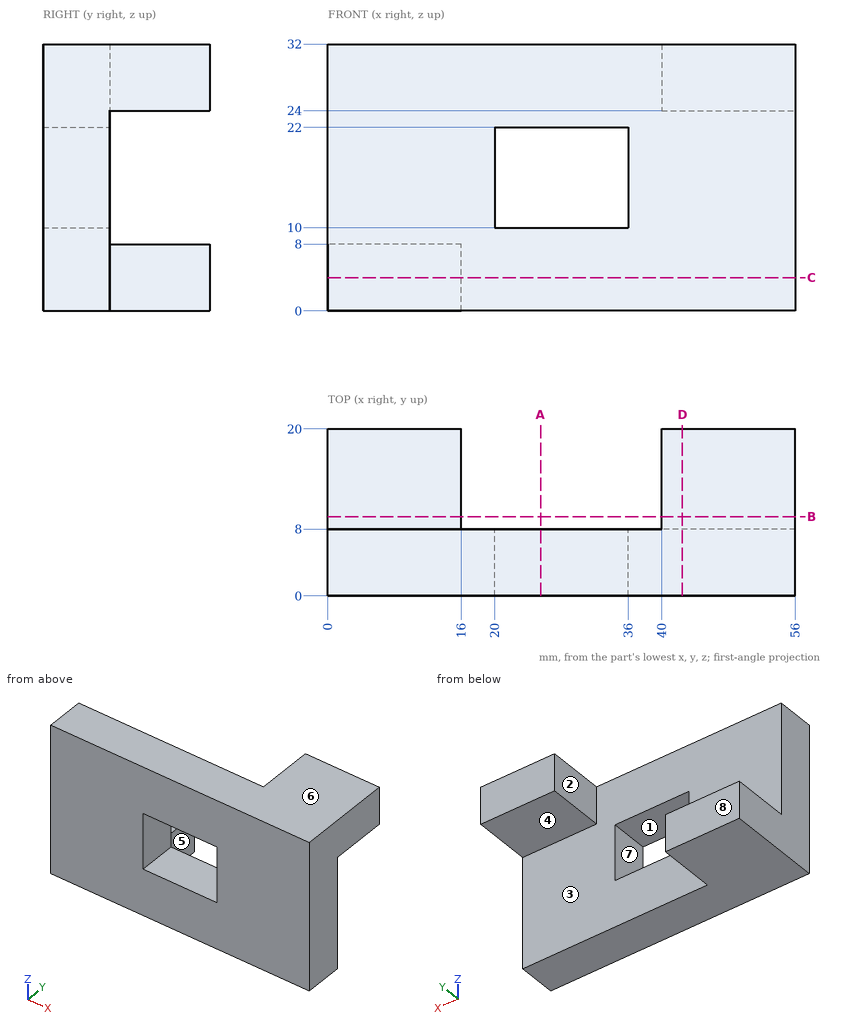
The drawing under review shows one solid part. Ordinate dimensions are in mm from its lowest x, y, z. A direction names the side the tool comes from. Coordinates: 2 decimals unless noted, no trailing zeros. Loops run counter-clockwise (first coordinate to the right, second up) from the corner with the lowest first, then second, coordinate; pieces in that order, holes last. Notation, with made-up numbers: (-37.5, -30) - (14.5, -30) arc R18 ccw to (14.5, -23) - close; hole circle Ø9 at (3, -9). An arc over 180 degrees is marked (long way). Return JSON: item names as keys, results as strings.
Item 1: Mouldability with a two-part tool opening along X and no side actions: class the marked faces 1, 2 and 3 as pulls with the +X half, pulls with the -X half, needs draft (parallel to the pull), parting line crosses it, or undercut.
Determined:
{"face 1": "undercut", "face 2": "pulls with the -X half", "face 3": "needs draft"}
Item 2: Take a section at B-B (y = 9.5). Give the boundary of the cut face in (x, z), then the cut area to 3 significant figures.
Determined:
{"outline": "(0, 0) - (16, 0) - (16, 8) - (0, 8) - close; (40, 24) - (56, 24) - (56, 32) - (40, 32) - close", "area": "256 mm2"}
Item 3: Take a section at C-C (z = 4). Give the boundary of the cut face in (x, y).
Determined:
{"outline": "(0, 0) - (56, 0) - (56, 8) - (16, 8) - (16, 20) - (0, 20) - close"}
Item 4: For the marked faces 4, 5, 6, 7 and 8, list the 3-axis set-ups (+Z, -Z, +X, -X, +Y, -Y) from which the entire face can be reached by the end or side of a thin tool; tool diameter is ignored.
Determined:
{"face 4": "-Z, +X, -X, +Y", "face 5": "+Z, -Z, +X, +Y", "face 6": "+Z, +X, -X, +Y, -Y", "face 7": "+Y, -Y", "face 8": "+Z, -Z, +X, -X, +Y"}
Item 5: Insertion check: pin 1 (6.5 mm diameter, centred on y = 16, z = 29, fed in from -X); pin 2 (9.5 mm diameter, centred on x = 5, y = 13, fed in from +Z); pin 3 (10 mm diameter, centred on y = 16, z = 13.5, fed in from -X); pin 4 (4 mm diameter, centred on x = 32.5, z = 23, fed in from +Y). Each pin has a flat end and moves straight along its axis. Give the tip position at first contact, or say it passes through.
Determined:
{"pin 1": "stops at x = 40", "pin 2": "stops at z = 8", "pin 3": "passes through", "pin 4": "stops at y = 8"}
Item 6: For line 1 (Z direction, x = 46, y = 18); line 2 (Z direction, x = 10, y = 15); line 3 (Z direction, x = 27, y = 7), list the stretches that pass through material, from the lowest coordinate up.
Determined:
{"line 1": "z = 24 to 32", "line 2": "z = 0 to 8", "line 3": "z = 0 to 10, 22 to 32"}
Item 7: Take a section at D-D (x = 42.5). Give the boundary of the cut face in (y, z).
Determined:
{"outline": "(0, 0) - (8, 0) - (8, 24) - (20, 24) - (20, 32) - (0, 32) - close"}
Item 8: Take a section at A-A (x = 25.5). Give the boundary of the cut face in (y, z).
Determined:
{"outline": "(0, 0) - (8, 0) - (8, 10) - (0, 10) - close; (0, 22) - (8, 22) - (8, 32) - (0, 32) - close"}
